Answer from the drawing. Dimensions are ordinates in mm from the lowest x, y and z of the part. A direction names the side the tool comes from. Coordinates: 2 decimals unless noted, no trailing zeros. Write each loop counter-clockwise with the first axis right and the second up, starting at its lowest first coordinate (ties: lowest second). Pieces come first, ordered by that corner, then holes.
(1) The part is cut by section A-A on y = 6. Determine the outline of the cut face in (x, z).
(2) The part is cut by section C-C on z = 9.75. Determine the outline of the cut face in (x, y), plus the area to 3 significant figures.
(3) Which of the six approach directions +Z, -Z, +X, -X, +Y, -Y give full straight-line access (tool end or side, diameter ignored) to the marked faces 1 and 2?
(4) The part is cut by section B-B on x = 15. Determine the outline of the cut face in (y, z), plus the area to 3 significant figures.
(5) For a pull along Z with two mould halves and no side action, classify the marked faces 3, 4 and 5 as +Z half, -Z half, draft (parallel to the pull), parting line (faces both ways), or undercut.
(6) A straight line is drawn through the part: line 1 (Z direction, x = 14.25, y = 3.75). Find the intervals that lie inside material, in ascending order.
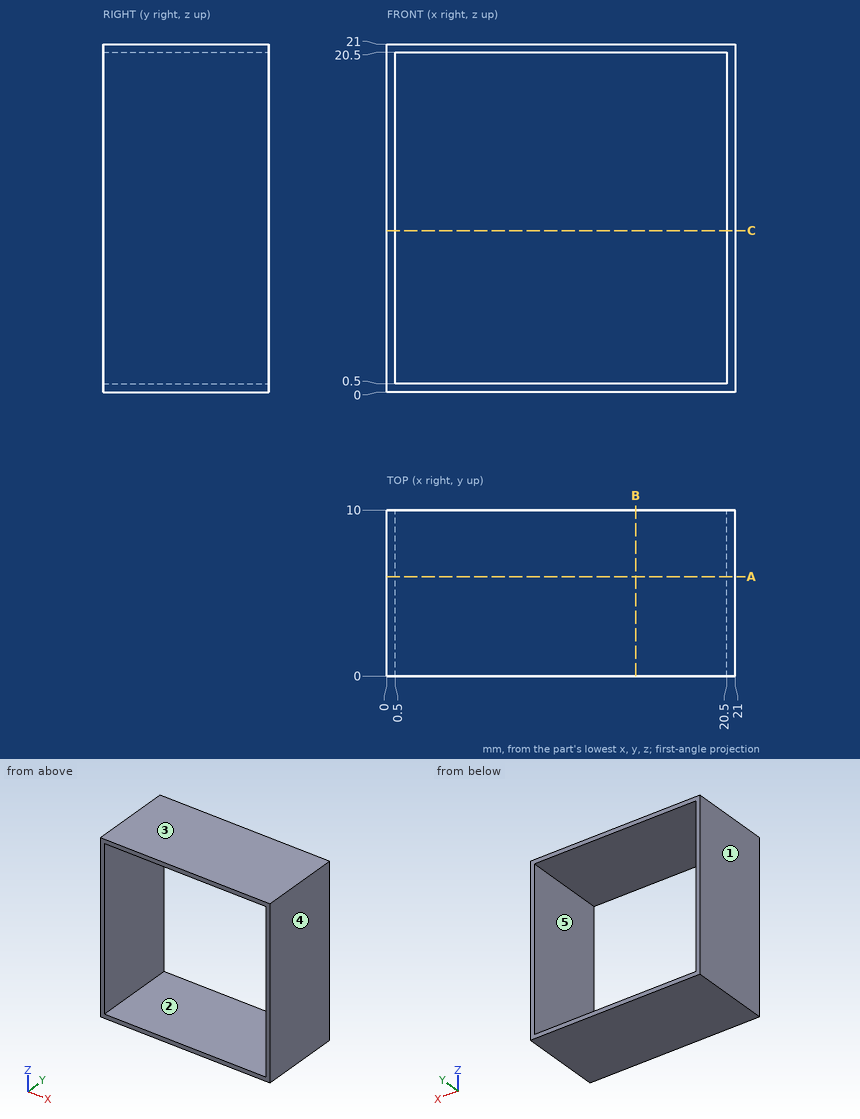
Model answer:
1. outline: (0, 0) - (21, 0) - (21, 21) - (0, 21) - close; hole (0.5, 0.5) - (20.5, 0.5) - (20.5, 20.5) - (0.5, 20.5) - close
2. outline: (0, 0) - (0.5, 0) - (0.5, 10) - (0, 10) - close; (20.5, 0) - (21, 0) - (21, 10) - (20.5, 10) - close
2. area: 10.0 mm2
3. face 1: +Z, -Z, -X, +Y, -Y
3. face 2: +Y, -Y
4. outline: (0, 0) - (10, 0) - (10, 0.5) - (0, 0.5) - close; (0, 20.5) - (10, 20.5) - (10, 21) - (0, 21) - close
4. area: 10.0 mm2
5. face 3: +Z half
5. face 4: draft
5. face 5: undercut
6. line 1: z = 0 to 0.5, 20.5 to 21
